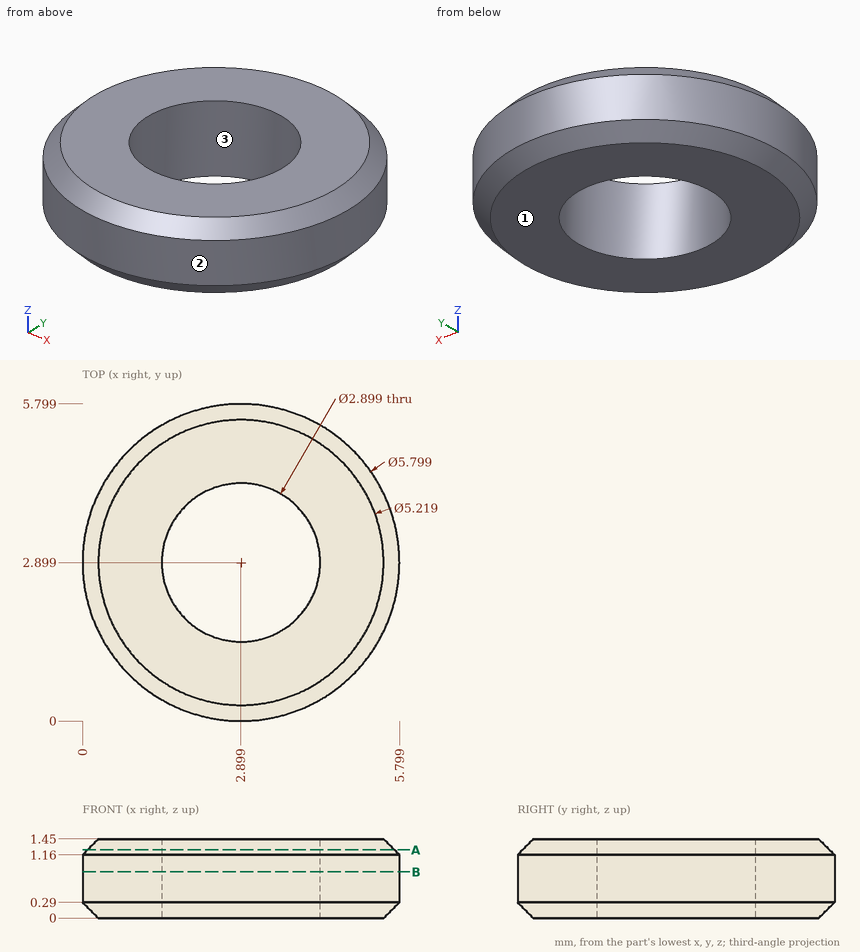
Study the drawing (mm; zero at the part's minimum x, y, z) and answer. Round coordinates to 2 decimals unless told otherwise and drop trailing zeros. Write each loop counter-clockwise with the first axis right and the second up, starting at its lowest first coordinate (ties: lowest second). Pieces come first, ordered by that corner, then holes. Notation, with made-up numbers: (59.5, 63) - (82.5, 63) arc R21 ccw to (82.5, 78) - close; hole circle Ø2 at (29, -33). An arc over 180 degrees is marked (long way). Use a Markdown table: item, result. Add a question column.
1. The part is cut by section A-A (z = 1.25). Write down the section's boundary in (x, y), and give its area (3 significant figures).
2. The part is cut by section B-B (z = 0.85). Write down the section's boundary in (x, y).
3. For a pull along Y with two mould halves and no side action, classify the marked faces 1, 2 and 3 as +Y half, -Y half, draft (parallel to the pull), parting line (faces both ways), or undercut.
4. Consider line 1 (Y direction, x = 3.9, z = 0.75); line 2 (X direction, y = 2.45, z = 0.25) (1 decimal); line 3 (Y direction, x = 3.45, z = 0.8) (1 decimal). Determine where each line is inside the solid, lowest interval first.
Reported:
| question | item | result |
|---|---|---|
| 1 | outline | circle Ø5.62 at (2.9, 2.9); hole circle Ø2.9 at (2.9, 2.9) |
| 1 | area | 18.2 mm^2 |
| 2 | outline | circle Ø5.8 at (2.9, 2.9); hole circle Ø2.9 at (2.9, 2.9) |
| 3 | face 1 | draft |
| 3 | face 2 | parting line |
| 3 | face 3 | undercut |
| 4 | line 1 | 0.18 to 1.85, 3.95 to 5.62 |
| 4 | line 2 | 0.1 to 1.5, 4.3 to 5.7 |
| 4 | line 3 | 0.1 to 1.6, 4.2 to 5.7 |
